Can you work these out from the model? Positions are in its coordinate system, mm. Face numbers are marked on the shaded views. A direction names the side the tool comes from. Coordinates: 2 decimals unless noted, no trailing zeros. Loops run counter-clockwise (first coordinate to the right, second up) from the corner with the lowest first, then second, coordinate; pieces in that order, holes last.
```python
from build123d import *

# Parameters (mm, degrees)
F0_W      = 1440
F0_H      = 800
F1_DEPTH  = 500
F3_DEPTH  = 400
F5_DEPTH  = 400
F7_DEPTH  = 100.001
F9_DEPTH  = 100.001
F10_W     = 900
F10_H     = 420
F11_DEPTH = 150
F12_R     = 40
F13_R     = 80
F14_DEPTH = 150
F15_R     = 80
F16_DEPTH = 500.001


with BuildPart() as f1:
    # F0 (on Front) → F1 (new body)
    with BuildSketch(Plane.XZ):
        Rectangle(F0_W, F0_H)
    extrude(amount=F1_DEPTH)

    # F2 (on face) → F3 (cut)
    with BuildSketch(Plane.XZ.offset(500)):
        with BuildLine():
            Line((280, 140), (-280, 140))
            ThreePointArc((-280, 140), (-308.2842712475, 128.2842712475), (-320, 100))
            Line((-320, 100), (-320, -210))
            ThreePointArc((-320, -210), (-308.2842712475, -238.2842712475), (-280, -250))
            Line((-280, -250), (280, -250))
            ThreePointArc((280, -250), (308.2842712475, -238.2842712475), (320, -210))
            Line((320, -210), (320, 100))
            ThreePointArc((320, 100), (308.2842712475, 128.2842712475), (280, 140))
        make_face()
    extrude(amount=-F3_DEPTH, mode=Mode.SUBTRACT)

    # F4 (on face) → F5 (cut)
    with BuildSketch(Plane.XZ.offset(500)):
        with BuildLine():
            Line((-720, 400), (-720, -270))
            Line((-720, -270), (-540, -270))
            ThreePointArc((-540, -270), (-511.7157287525, -258.2842712475), (-500, -230))
            Line((-500, -230), (-500, 400))
            Line((-500, 400), (-720, 400))
        make_face()
        with BuildLine():
            Line((720, 400), (500, 400))
            Line((500, 400), (500, -230))
            ThreePointArc((500, -230), (511.7157287525, -258.2842712475), (540, -270))
            Line((540, -270), (720, -270))
            Line((720, -270), (720, 400))
        make_face()
    extrude(amount=-F5_DEPTH, mode=Mode.SUBTRACT)

    # F6 (on face) → F7 (cut, through all)
    with BuildSketch(Plane.XZ.offset(100)):
        Polygon((500, 400), (720, -30), (720, 400), align=None)
    extrude(amount=-F7_DEPTH, mode=Mode.SUBTRACT)

    # F8 (on face) → F9 (cut, through all)
    with BuildSketch(Plane.XZ.offset(100)):
        Polygon((-720, 400), (-720, -30), (-500, 400), align=None)
    extrude(amount=-F9_DEPTH, mode=Mode.SUBTRACT)

    # F10 (on face) → F11 (cut)
    with BuildSketch(Plane.XY.offset(400)):
        with Locations((0, -290)):
            Rectangle(F10_W, F10_H)
    extrude(amount=-F11_DEPTH, mode=Mode.SUBTRACT)

    # F12
    f12_edges = [f1.edges().sort_by_distance(p)[0] for p in [
        (-450, -290, 250),
        (450, -290, 250),
    ]]
    fillet(f12_edges, radius=F12_R)

    # F13 (on face) → F14 (cut)
    with BuildSketch(Plane.XY.offset(250)):
        with Locations((0, -290)):
            Circle(F13_R)
    extrude(amount=-F14_DEPTH, mode=Mode.SUBTRACT)

    # F15 (on face) → F16 (cut, through all)
    with BuildSketch(Plane(origin=(0, 0, 0), x_dir=(-1, 0, 0), z_dir=(0, 1, 0))):
        with Locations((0, -55)):
            Circle(F15_R)
    extrude(amount=-F16_DEPTH, mode=Mode.SUBTRACT)


solid = f1.part
```
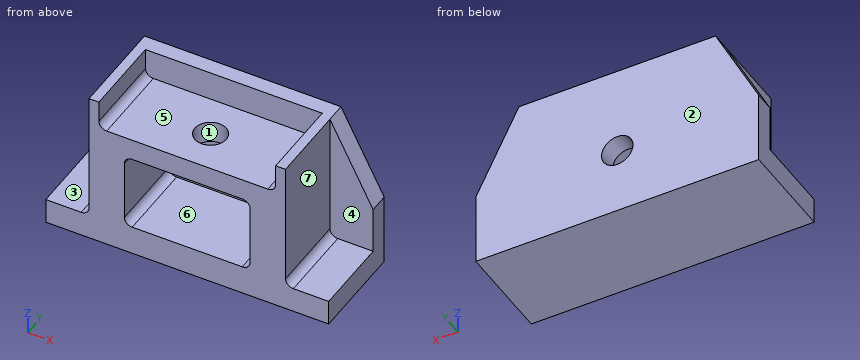
(1) I want a section at B-B on x = 0. Write out the boundary of the cut face in (y, z), then the cut area to 3 significant figures.
Check values:
outline: (-500, -400) - (0, -400) - (0, -135) - (-100, -135) - (-100, -250) - (-500, -250) - close; (-500, 140) - (-370, 140) - (-370, 250) - (-500, 250) - close; (-210, 140) - (-100, 140) - (-100, 25) - (0, 25) - (0, 400) - (-80, 400) - (-80, 250) - (-210, 250) - close
area: 147,000 mm2
(2) I want a section at A-A on z = -55. Write out the boundary of the cut face in (x, y).
Check values:
outline: (-720, -100) - (-500, -100) - (-500, -500) - (-320, -500) - (-320, -100) - (-80, -100) - (-80, 0) - (-720, 0) - close; (80, -100) - (320, -100) - (320, -500) - (500, -500) - (500, -100) - (720, -100) - (720, 0) - (80, 0) - close
(3) I'm going to push flat-ended pins straight in: pin 1 (2 mm diameter, centred on y = -245, z = 123.5, fed in from -X); pin 2 (10 mm diameter, centred on y = -299, z = 313.5, fed in from +X); pin 3 (1.5 mm diameter, centred on x = 66.5, y = -115, fed in from +Z). Where does each tip first touch, or does it pass through?
Check values:
pin 1: stops at x = -500
pin 2: stops at x = 500
pin 3: stops at z = 250
(4) Which directions (+Z, -Z, +X, -X, +Y, -Y) give clear straight access to the entire face, cutting with the end or side of a thin tool? Please do the marked faces 5, 6 and 7.
Check values:
face 5: +Z, -Y
face 6: -Y
face 7: +Z, +X, -Y
(5) If we mould it in two halves opening along Y, with no side actions, what happens to the marked faces 1, 2, 3 and 4? For each: released by +Y, released by -Y, zero draft, split by the parting line, or undercut.
Check values:
face 1: undercut
face 2: released by +Y
face 3: zero draft
face 4: released by -Y
(6) I want a section at D-D on x = 393. Write out the boundary of the cut face in (y, z).
Check values:
outline: (-500, -400) - (0, -400) - (0, 400) - (-80, 400) - (-80, 250) - (-500, 250) - close
(7) If I drill on probe 1 along X at (y, z) = (-310.5, 353); probe 2 along Z at (x, y) = (0, -54); probe 3 along Z at (x, y) = (162, -433.5), over which ranges is the centre line in solid material (lowest first)?
Check values:
probe 1: x = -500 to -450, 450 to 500
probe 2: z = -400 to -135, 25 to 400
probe 3: z = -400 to -250, 140 to 250
(8) I want a section at C-C on y = -192. Write out the boundary of the cut face in (x, z).
Check values:
outline: (-720, -400) - (720, -400) - (720, -270) - (540, -270) arc R40 cw to (500, -230) - (500, 400) - (450, 400) - (450, 290) arc R40 cw to (410, 250) - (-410, 250) arc R40 cw to (-450, 290) - (-450, 400) - (-500, 400) - (-500, -230) arc R40 cw to (-540, -270) - (-720, -270) - close; hole (-320, -210) arc R40 ccw to (-280, -250) - (280, -250) arc R40 ccw to (320, -210) - (320, 100) arc R40 ccw to (280, 140) - (-280, 140) arc R40 ccw to (-320, 100) - close
